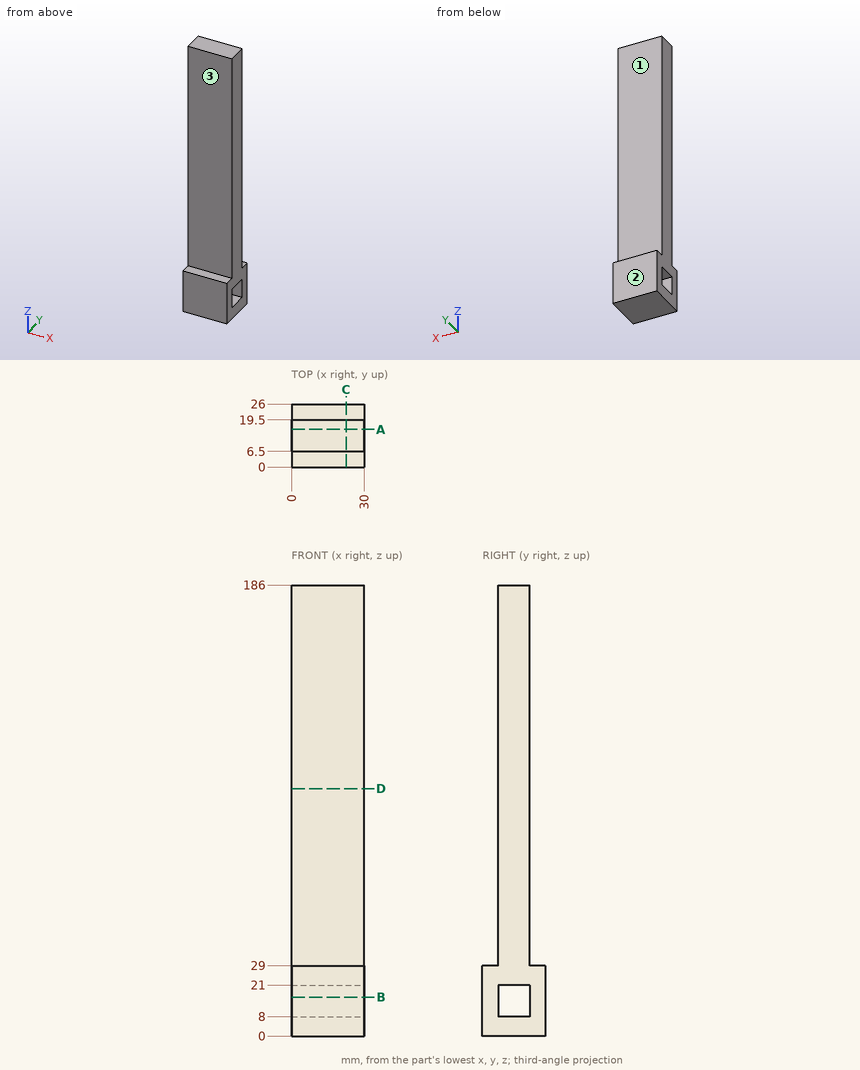
Study the drawing (mm; zero at the part's minimum x, y, z) and answer. A direction names the side the tool comes from. Coordinates: 2 decimals unless noted, no trailing zeros. Write each loop counter-clockwise with the first axis right and the second up, starting at its lowest first coordinate (ties: lowest second). Pieces come first, ordered by that corner, then holes. Notation, with made-up numbers: (-9.5, -20.75) - (13.5, -20.75) arc R17 cw to (13.5, 9.25) - close; hole circle Ø1 at (69.5, 37). An arc over 180 degrees is marked (long way). Put each result on its own line as item: value.
1. Flat-ended cylindrical pins translate along their axes: pin 1 Ø4 at (x, z) = (13.5, 136.5) entering from -Y; pin 2 Ø1 at (x, z) = (18.5, 25.5) entering from -Y; pin 3 Ø1.5 at (x, z) = (25.5, 131.5) entering from +Y; pin 4 Ø5 at (x, y) = (12, 22.5) entering from +Z. Find the tip coordinate at first contact, or state that the pin passes through.
Answer sheet:
pin 1: stops at y = 6.5
pin 2: stops at y = 0
pin 3: stops at y = 19.5
pin 4: stops at z = 29
2. The part is cut by section C-C on x = 22.5. Give the vertices of the cut face in (y, z).
Answer sheet:
outline: (0, 0) - (26, 0) - (26, 29) - (19.5, 29) - (19.5, 186) - (6.5, 186) - (6.5, 29) - (0, 29) - close; hole (6.5, 8) - (19.5, 8) - (19.5, 21) - (6.5, 21) - close
3. The part is cut by section D-D on z = 102. Give the vertices of the cut face in (x, y).
Answer sheet:
outline: (0, 6.5) - (30, 6.5) - (30, 19.5) - (0, 19.5) - close
4. A tool of negligible diameter and unlimited length cuts with its end or side. For the marked faces 1, 2 and 3, from which of +Z, -Z, +X, -X, +Y, -Y can it reach the whole face along a straight path? Write none if from no direction.
Answer sheet:
face 1: +Z, +X, -X, +Y
face 2: +Z, -Z, +X, -X, +Y
face 3: +Z, +X, -X, -Y
5. The part is cut by section B-B on z = 16. Give the vertices of the cut face in (x, y).
Answer sheet:
outline: (0, 0) - (30, 0) - (30, 6.5) - (0, 6.5) - close; (0, 19.5) - (30, 19.5) - (30, 26) - (0, 26) - close
6. Find the intervals of material crossed by line 1 along Z through (x, y) = (13.5, 14.75); line 2 along Y through (x, z) = (4.75, 40); line 3 along Y through (x, z) = (21.75, 9), in increasing order. Write a range as from..to.
Answer sheet:
line 1: z = 0..8, 21..186
line 2: y = 6.5..19.5
line 3: y = 0..6.5, 19.5..26
7. The part is cut by section A-A on y = 15.5. Give the vertices of the cut face in (x, z), plus the area to 3 significant figures.
Answer sheet:
outline: (0, 0) - (30, 0) - (30, 8) - (0, 8) - close; (0, 21) - (30, 21) - (30, 186) - (0, 186) - close
area: 5,190 mm^2
